from build123d import *

# Parameters (mm, degrees)
SKETCH_1_W                       = 450
SKETCH_1_H                       = 210
EXTRUDE_797_DEPTH                = 5
SKETCH_2_W                       = 40
SKETCH_2_H                       = 10
EXTRUDE_849_DEPTH                = 5
CHAMFER_897_SIZE                 = 1.5
SKETCH_3_W                       = 40
SKETCH_3_H                       = 10
EXTRUDE_968_DEPTH                = 5
CHAMFER_1013_SIZE                = 1.5
CHAMFER_1013_OF_MIRROR_1076_SIZE = 1.5
MIRROR_START                     = -5
MIRROR_1098_DEPTH                = 10
HOLE_WIZARD_1123_D               = 5.5
HOLE_WIZARD_1123_DEPTH           = 10
HOLE_WIZARD_1123_TIP             = 1.652366702


# Read off the part's stored shape, not the designer's step: ほぞ(左)
with BuildPart() as part:
    # ｽｹｯﾁ1 → Extrude 797 (new, symmetric)
    with BuildSketch(Plane(origin=(0, 0, 0), x_dir=(1, 0, 0), z_dir=(0, 1, 0))):
        Rectangle(SKETCH_1_W, SKETCH_1_H)
    extrude(amount=EXTRUDE_797_DEPTH, both=True)

    # ｽｹｯﾁ2 → Extrude 849 (add, symmetric)
    with BuildSketch(Plane(origin=(0, 0, 0), x_dir=(1, 0, 0), z_dir=(0, 1, 0))):
        with Locations((0, -110)):
            Rectangle(SKETCH_2_W, SKETCH_2_H)
    extrude(amount=EXTRUDE_849_DEPTH, both=True)

    # Chamfer 897
    chamfer_897_edges = [part.edges().sort_by_distance(p)[0] for p in [
        (-20, 0, 115),
        (20, 0, 115),
    ]]
    chamfer(chamfer_897_edges, length=CHAMFER_897_SIZE)

    # ｽｹｯﾁ3 → Extrude 968 (add, symmetric)
    with BuildSketch(Plane(origin=(0, 0, 0), x_dir=(1, 0, 0), z_dir=(0, 1, 0))):
        with Locations((170, -110)):
            Rectangle(SKETCH_3_W, SKETCH_3_H)
    extrude_968 = extrude(amount=EXTRUDE_968_DEPTH, both=True)

    # Chamfer 1013
    chamfer_1013_edges = [part.edges().sort_by_distance(p)[0] for p in [
        (150, 0, 115),
        (190, 0, 115),
    ]]
    chamfer(chamfer_1013_edges, length=CHAMFER_1013_SIZE)

    # Mirror 1076: Extrude 968 across plane
    add(extrude_968.mirror(Plane(origin=(0, 0, 0), x_dir=(0, 0, 1), z_dir=(1, 0, 0))))

    # Chamfer 1013 of Mirror 1076
    chamfer_1013_of_mirror_1076_edges = [part.edges().sort_by_distance(p)[0] for p in [
        (-150, 0, 115),
        (-190, 0, 115),
    ]]
    chamfer(chamfer_1013_of_mirror_1076_edges, length=CHAMFER_1013_OF_MIRROR_1076_SIZE)

    # Mirror 1098 outline → Mirror 1098 (add)
    with BuildSketch(Plane(origin=(0, 0, 0), x_dir=(1, 0, 0), z_dir=(0, 1, 0)).offset(MIRROR_START)):
        Polygon((-18.5, 115), (-20, 113.5), (-20, 105), (20, 105), (20, 113.5), (18.5, 115), align=None)
        Polygon((150, 113.5), (150, 105), (190, 105), (190, 113.5), (188.5, 115), (151.5, 115), align=None)
        Polygon((-190, 105), (-150, 105), (-150, 113.5), (-151.5, 115), (-188.5, 115), (-190, 113.5), align=None)
    extrude(amount=MIRROR_1098_DEPTH)

    # Hole Wizard 1123
    with Locations(Plane(origin=(0, 5, 0), x_dir=(1, 0, 0), z_dir=(0, 1, 0))):
        with Locations((100, -13), (100, 13), (62, -13), (62, 13)):
            Hole(HOLE_WIZARD_1123_D / 2, depth=HOLE_WIZARD_1123_DEPTH)
            with Locations((0, 0, -(HOLE_WIZARD_1123_DEPTH + HOLE_WIZARD_1123_TIP / 2))):  # 118° drill point
                Cone(0, HOLE_WIZARD_1123_D / 2, HOLE_WIZARD_1123_TIP, mode=Mode.SUBTRACT)


solid = part.part
Could you check a few things on this model? Use its own coordinates, in mm. A direction names the side the tool comes from. Give positions to 0.01 mm unless a question says otherwise; leave off trailing zeros. Write each loop counter-clockwise with the first axis right and the second up, starting at its lowest first coordinate (ties: lowest second). Pieces come first, ordered by that corner, then holes. Notation, with made-up numbers: (56, 29.5) -> (73, 29.5) arc R31 ccw to (73, 54.5) -> close; hole circle Ø8 at (6, -33.75). An arc over 180 degrees is marked (long way). Answer as CSV lines item,"result". Start each with the question number.
(1) If we section it at A-A, the plane x = 133: Write out the boundary of the cut face in (y, z), and give its area (3 significant figures).
(2) If we section it at B-B, the plane y = -3.25: Give the number of separate pieces and of enclosed holes in the cut face, and give its area (3 significant figures).
(3) I'm going to push flat-ended pins straight in: pin 1 Ø5 at (x, y) = (-214.5, 1) entering from +Z; pin 2 Ø4.5 at (y, z) = (0.5, 111) entering from +X; pin 3 Ø5 at (x, y) = (-102.5, 0.5) entering from -Z. Where does each tip first touch, or does it pass through?
(4) Please list where these lines run through material, in increasing order: line 1 (X direction, y = -1, z = -13); line 2 (Z direction, x = 62, y = 2.25); line 3 (Z direction, x = 135, y = -4.25).
(5) Which directions (+Z, -Z, +X, -X, +Y, -Y) give clear straight access to the entire face, cutting with the end or side of a thin tool? Please do faces 1 (the face through (-20, 0, 109)), 2 (the face through (-208, 0, 105)), 3 (the face through (-190, 0, -109)), 4 (the face through (150, 0, -109)), 5 (the face through (190, 0, -109)).
Answer list:
1,outline,"(-5, -105) -> (5, -105) -> (5, 105) -> (-5, 105) -> close"
1,area,"2,100 mm^2"
2,separate pieces,"1"
2,enclosed holes,"4"
2,area,"96,800 mm^2"
3,pin 1,"z = 105"
3,pin 2,"x = 190"
3,pin 3,"z = -105"
4,line 1,"-225 to 59.25, 64.75 to 97.25, 102.75 to 225"
4,line 2,"-105 to -15.75, -10.25 to 10.25, 15.75 to 105"
4,line 3,"-105 to 105"
5,face 1,"+Z, +Y, -Y"
5,face 2,"+Z, -X, +Y, -Y"
5,face 3,"-Z, -X, +Y, -Y"
5,face 4,"-Z, +Y, -Y"
5,face 5,"-Z, +X, +Y, -Y"
